Verification items for the finished model (mm, model axes). Face numbers are marked on the shaded views. A direction names the side the tool comes from. Coordinates: 2 decimals unless noted, no trailing zeros. Write each loop counter-clockwise with the first axis right and the second up, starting at its lowest first coordinate (ties: lowest second). Pieces come first, ordered by that corner, then holes. Notation, with made-up numbers: (-3, 68.5) - (54, 68.5) arc R26 cw to (54, 98.5) - close; hole circle Ø9 at (79, 89). An arc over 180 degrees is marked (long way). Use one line per item in the form item = value. Start each with the question number.
(1) Tool access check on the marked faces 1 and 2. Record the directions out of +Z, -Z, +X, -X, +Y, -Y that give a thin tool (end or side, any length) a straight path to the whole face; none if there is none.
(2) Sectioned sample at B-B (x = 7). Record the cut outline in (y, z), and give its area (3 significant figures).
(3) Gauge pin test, flat ends, axial feed: pin 1 Ø6.5 at (x, y) = (0, 0) entering from +Z; pin 2 Ø2 at (x, y) = (5, 6.5) entering from +Z; pin 3 Ø3.5 at (x, y) = (0, 0) entering from +Z. Record the tip position at first contact, or that the pin passes through.
(4) Mould release check, pull along Y, two halves, no side actions. Record for the marked faces 3, 4 and 5: released by +Y, released by -Y, zero draft, split by the parting line, or undercut.
(5) Material ranges on line 1 (Y direction, x = 0, z = 0.5); line 2 (Y direction, x = 0, z = 2.45); line 3 (Z direction, x = 7, y = 1.25), recorded low to high. Write a range as [from, to].
(6) Sectioned sample at A-A (y = 0). Record the cut outline in (x, z).
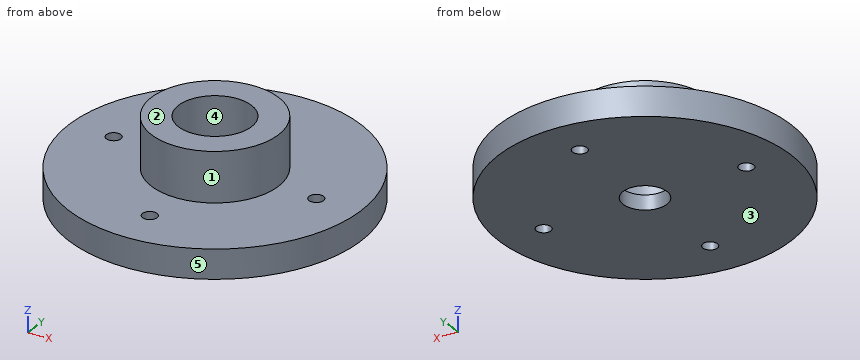
from build123d import *

# Parameters (mm, degrees)
SKETCH_1_R          = 10
EXTRUDE_1_DEPTH     = 2
SKETCH_2_R          = 4.35
EXTRUDE_2_DEPTH     = 3.4
SKETCH_3_R          = 1.5
CUT_EXTRUDE_1_DEPTH = 9.4
SKETCH_4_R          = 0.5
CUT_EXTRUDE_3_DEPTH = 16.4
SKETCH_5_R          = 2.5
CUT_EXTRUDE_4_DEPTH = 4.4


with BuildPart() as part:
    # 草图1 → 凸台-拉伸1 (new body)
    with BuildSketch(Plane.XY):
        Circle(SKETCH_1_R)
    extrude(amount=EXTRUDE_1_DEPTH)

    # 草图2 → 凸台-拉伸2 (add)
    with BuildSketch(Plane.XY.offset(2)):
        Circle(SKETCH_2_R)
    extrude(amount=EXTRUDE_2_DEPTH)

    # 草图3 → 切除-拉伸1 (cut)
    with BuildSketch(Plane.XY):
        Circle(SKETCH_3_R)
    extrude(amount=CUT_EXTRUDE_1_DEPTH, mode=Mode.SUBTRACT)

    # 草图4 → 切除-拉伸3 (cut)
    with BuildSketch(Plane.XY):
        with Locations((0, 7)):
            Circle(SKETCH_4_R)
        with Locations((7, 0)):
            Circle(SKETCH_4_R)
        with Locations((0, -7)):
            Circle(SKETCH_4_R)
        with Locations((-7, 0)):
            Circle(SKETCH_4_R)
    extrude(amount=CUT_EXTRUDE_3_DEPTH, mode=Mode.SUBTRACT)

    # 草图5 → 切除-拉伸4 (cut)
    with BuildSketch(Plane.XY.offset(5.4)):
        Circle(SKETCH_5_R)
    extrude(amount=-CUT_EXTRUDE_4_DEPTH, mode=Mode.SUBTRACT)


solid = part.part
Answers below:
q1.face_1 = +Z
q1.face_2 = +Z, +X, -X, +Y, -Y
q2.outline = (-7.14, 0) - (-0.5, 0) - (-0.5, 2) - (-7.14, 2) - close; (0.5, 0) - (7.14, 0) - (7.14, 2) - (0.5, 2) - close
q2.area = 26.6 mm2
q3.pin_1 = 5.4
q3.pin_2 = 2
q3.pin_3 = 1
q4.face_3 = zero draft
q4.face_4 = undercut
q4.face_5 = split by the parting line
q5.line_1 = [-10, -7.5], [-6.5, -1.5], [1.5, 6.5], [7.5, 10]
q5.line_2 = [-4.35, -2.5], [2.5, 4.35]
q5.line_3 = [0, 2]
q6.outline = (-10, 0) - (-7.5, 0) - (-7.5, 2) - (-10, 2) - close; (-6.5, 0) - (-1.5, 0) - (-1.5, 1) - (-2.5, 1) - (-2.5, 5.4) - (-4.35, 5.4) - (-4.35, 2) - (-6.5, 2) - close; (1.5, 0) - (6.5, 0) - (6.5, 2) - (4.35, 2) - (4.35, 5.4) - (2.5, 5.4) - (2.5, 1) - (1.5, 1) - close; (7.5, 0) - (10, 0) - (10, 2) - (7.5, 2) - close
